Verification items for the finished model (mm, model axes). A direction names the side the tool comes from. Coordinates: 2 decimals unless noted, no trailing zeros. Loops run counter-clockwise (first coordinate to the right, second up) from the corner with the lowest first, then second, coordinate; pieces in that order, holes last.
Q1. Access from +Z, -Z, +X, -X, +Y, -Y to the whole of each face (thin tool, end or side, straight path). Record for faces 5 (the face through (-64.31, -64, 1.48)), 6 (the face through (-85.8, -89, 4)), 7 (the face through (-63, -78, 4)), 8 (the face through (-61.7, -66.3, 3)), 9 (the face through (-60, -79, 4)).
Q2. Go/stop test with flat-tipped pins: P1, Ø1.5, axis at x = -74, z = 6.5, coming from the +Y side; P2, Ø1.5, axis at x = -61.5, z = 6, coming from the +Y side; P3, Ø1.7, axis at y = -88.5, z = 4.5, coming from the -X side. Record where each tip stops, or that it passes through.
Q3. Sectioned sample at C-C (x = -69). Enter the section's corners in (y, z).
Q4. Mould release check, pull along Y, two halves, no side actions. Record for faces 1 (the face through (-62, -62, 1)), 2 (the face through (-66, -65, 1)), 3 (the face through (-75, -90, 4)), 4 (the face through (-87, -88.5, 2.4)): +Y half, -Y half, draft (parallel to the pull), parting line (faces both ways), or undercut.
Q5. Sectioned sample at B-B (z = 1.75). Enter the section's corners in (x, y).
Q6. Sectioned sample at A-A (y = -65). Enter the section's corners in (x, z), then the cut area to 3 significant figures.
Q7. Material ranges on probe 1 along X at (y, z) = (-65, 1.5); probe 2 along Y at (x, z) = (-64.5, 1.25); probe 3 along X at (y, z) = (-85.5, 3.25), recorded low to high.
Q8. Sectioned sample at D-D (y = -71). Enter the section's corners in (x, z), then the cut area to 3 significant figures.
Autodesk Inventor part; units mm, degrees
ref_plane "YZ Plane" through (0, 0, 0) normal (1, 0, 0) x (0, 1, 0)
ref_plane "XZ Plane" through (0, 0, 0) normal (0, 1, 0) x (-1, 0, 0)
ref_plane "XY Plane" through (0, 0, 0) normal (0, 0, 1) x (1, 0, 0)
sketch "Sketch1" plane through (0, 0, 0) normal (0, 0, 1) x (1, 0, 0)
  line L0 (-58, -60) -> (-60, -60)
  line L1 (-60, -60) -> (-60, -39.5)
  line L2 (-60, -39.5) -> (-58, -39.5)
  line L3 (-58, -39.5) -> (-58, -60)
  line L4 (49.6, 30) -> (51.6, 30)
  line L5 (51.6, 30) -> (51.6, 9.5)
  line L6 (51.6, 9.5) -> (49.6, 9.5)
  line L7 (49.6, 9.5) -> (49.6, 30)
  line L8 (-58, 39.5) -> (-60, 39.5)
  line L9 (-60, 39.5) -> (-60, 60)
  line L10 (-60, 60) -> (-58, 60)
  line L11 (-58, 60) -> (-58, 39.5)
  line L12 (-21.6, -39.5) -> (-19.6, -39.5)
  line L13 (-19.6, -39.5) -> (-19.6, -60)
  line L14 (-19.6, -60) -> (-21.6, -60)
  line L15 (-21.6, -60) -> (-21.6, -39.5)
  line L16 (51.6, -30) -> (49.6, -30)
  line L17 (49.6, -30) -> (49.6, -9.5)
  line L18 (49.6, -9.5) -> (51.6, -9.5)
  line L19 (51.6, -9.5) -> (51.6, -30)
  line L20 (-21.6, 60) -> (-19.6, 60)
  line L21 (-19.6, 60) -> (-19.6, 39.5)
  line L22 (-19.6, 39.5) -> (-21.6, 39.5)
  line L23 (-21.6, 39.5) -> (-21.6, 60)
  line L24 (90, -35) -> (90, 35)
  line L25 (90, 35) -> (49.6, 35)
  line L26 (49.6, 35) -> (49.6, 60)
  line L27 (49.6, 60) -> (90, 60)
  line L28 (90, 60) -> (90, 90)
  line L29 (90, 90) -> (-19.6, 90)
  line L30 (-19.6, 90) -> (-19.6, 65)
  line L31 (-19.6, 65) -> (-60, 65)
  line L32 (-60, 65) -> (-60, 90)
  line L33 (-60, 90) -> (-90, 90)
  line L34 (-90, 90) -> (-90, -90)
  line L35 (-90, -90) -> (-60, -90)
  line L36 (-60, -90) -> (-60, -65)
  line L37 (-60, -65) -> (-19.6, -65)
  line L38 (-19.6, -65) -> (-19.6, -90)
  line L39 (-19.6, -90) -> (90, -90)
  line L40 (90, -90) -> (90, -60)
  line L41 (90, -60) -> (49.6, -60)
  line L42 (49.6, -60) -> (49.6, -35)
  line L43 (49.6, -35) -> (90, -35)
  line L44 (86, -32) -> (73.8, -32)
  line L45 (73.8, -32) -> (73.8, -7.5)
  line L46 (73.8, -7.5) -> (86, -7.5)
  line L47 (86, -7.5) -> (86, -32)
  line L48 (65.8, -32) -> (53.6, -32)
  line L49 (53.6, -32) -> (53.6, -7.5)
  line L50 (53.6, -7.5) -> (65.8, -7.5)
  line L51 (65.8, -7.5) -> (65.8, -32)
  line L52 (86, -86) -> (70.6, -86)
  line L53 (70.6, -86) -> (70.6, -69.8)
  line L54 (70.6, -69.8) -> (86, -69.8)
  line L55 (86, -69.8) -> (86, -86)
  line L56 (86, 86) -> (86, 69.8)
  line L57 (86, 69.8) -> (70.6, 69.8)
  line L58 (70.6, 69.8) -> (70.6, 86)
  line L59 (70.6, 86) -> (86, 86)
  line L60 (73.8, 32) -> (86, 32)
  line L61 (86, 32) -> (86, 7.5)
  line L62 (86, 7.5) -> (73.8, 7.5)
  line L63 (73.8, 7.5) -> (73.8, 32)
  line L64 (65.8, 32) -> (65.8, 7.5)
  line L65 (65.8, 7.5) -> (53.6, 7.5)
  line L66 (53.6, 7.5) -> (53.6, 32)
  line L67 (53.6, 32) -> (65.8, 32)
  line L68 (-69.6, -87) -> (-85, -87)
  line L69 (-85, -87) -> (-85, -70.8)
  line L70 (-85, -70.8) -> (-69.6, -70.8)
  line L71 (-69.6, -70.8) -> (-69.6, -87)
  line L72 (-56, -62) -> (-56, -37.5)
  line L73 (-56, -37.5) -> (-43.8, -37.5)
  line L74 (-43.8, -37.5) -> (-43.8, -62)
  line L75 (-43.8, -62) -> (-56, -62)
  line L76 (-56, 62) -> (-43.8, 62)
  line L77 (-43.8, 62) -> (-43.8, 37.5)
  line L78 (-43.8, 37.5) -> (-56, 37.5)
  line L79 (-56, 37.5) -> (-56, 62)
  line L80 (-23.6, 62) -> (-23.6, 37.5)
  line L81 (-23.6, 37.5) -> (-35.8, 37.5)
  line L82 (-35.8, 37.5) -> (-35.8, 62)
  line L83 (-35.8, 62) -> (-23.6, 62)
  line L84 (-23.6, -62) -> (-35.8, -62)
  line L85 (-35.8, -62) -> (-35.8, -37.5)
  line L86 (-35.8, -37.5) -> (-23.6, -37.5)
  line L87 (-23.6, -37.5) -> (-23.6, -62)
  line L88 (-85, 87) -> (-69.6, 87)
  line L89 (-69.6, 87) -> (-69.6, 70.8)
  line L90 (-69.6, 70.8) -> (-85, 70.8)
  line L91 (-85, 70.8) -> (-85, 87)
  line L92 (-63, -68) -> (-60, -68)
  line L93 (-60, -68) -> (-60, -65)
  line L94 (-60, -65) -> (-19.6, -65)
  line L95 (-90, -90) -> (-60, -90)
  line L96 (-60, -90) -> (-60, -87)
  line L97 (-60, -87) -> (-90, -87)
  line L98 (-90, -87) -> (-90, -90)
  line L99 (-60, -87) -> (-63, -87)
  line L100 (-63, -87) -> (-63, -68)
  line L101 (-63, -68) -> (-60, -68)
  line L102 (-60, -68) -> (-60, -87)
  line L103 (-60, -68) -> (-66, -68)
  line L104 (-66, -68) -> (-66, -62)
  line L105 (-66, -62) -> (-60, -62)
  line L106 (-60, -62) -> (-60, -68)
  circle A0 centre (-63, -65) radius 1.5
  circle A1 centre (-16.6, -87) radius 1.5
  circle A2 centre (49.6, -87) radius 1.5
  circle A3 centre (46.6, -60) radius 1.5
  circle A4 centre (87, -63) radius 1.5
  circle A5 centre (46.6, -32) radius 1.5
  circle A6 centre (46.6, 32) radius 1.5
  circle A7 centre (87, 63) radius 1.5
  circle A8 centre (46.6, 60) radius 1.5
  circle A9 centre (49.6, 87) radius 1.5
  circle A10 centre (-16.6, 87) radius 1.5
  circle A11 centre (-16.6, 65) radius 1.5
  circle A12 centre (-63, 65) radius 1.5
  arc A13 (-63, -62) -> (-63, -68) centre (-63, -65) ccw
  arc A14 (-16.6, -68) -> (-16.6, -62) centre (-16.6, -65) ccw
  line L107 (-16.6, -62) -> (-63, -62)
  line L108 (-76, -39.25) -> (-82, -39.25)
  line L109 (-82, -39.25) -> (-82, -20.75)
  line L110 (-82, -20.75) -> (-76, -20.75)
  line L111 (-76, -20.75) -> (-76, -39.25)
  line L112 (-76, 20.75) -> (-82, 20.75)
  line L113 (-82, 20.75) -> (-82, 39.25)
  line L114 (-82, 39.25) -> (-76, 39.25)
  line L115 (-76, 39.25) -> (-76, 20.75)
  line L116 (-19.6, -68) -> (-16.6, -68)
  circle A15 centre (-86.5, -55.7158) radius 1.25
  circle A16 centre (-86.5, 55.8) radius 1.25
  circle A17 centre (-79.5, -5.4579) radius 1.25
  circle A18 centre (-79.5, 5.5421) radius 1.25
  line L117 (-19.6, -65) -> (-19.6, -68)
  point P0 (0, 0)
  dimension "d0" = 3
extrude "Extrusion1" add sketch "Sketch1" along normal blind 8 contours L36 L97 L100 L92 | L36 L35 L34 L97 L68
ref_plane "Work Plane1" through (0, 0, 0) normal (0, 0, 1) x (1, 0, 0)
sketch "Sketch2" plane through (0, 0, 0) normal (0, 0, 1) x (1, 0, 0)
  line L0 (-63, -68) -> (-60, -68)
  line L1 (-60, -68) -> (-60, -65)
  line L2 (-60, -65) -> (-19.6, -65)
  circle A0 centre (-63, -65) radius 2
  line L3 (-60, -90) -> (-60, -68)
  line L4 (-60, -68) -> (-66, -68)
  line L5 (-66, -68) -> (-66, -62)
  line L6 (-66, -62) -> (-60, -62)
  line L7 (-60, -62) -> (-60, -68)
  circle A1 centre (-63, -65) radius 1.65
  arc A2 (-63, -62) -> (-63, -68) centre (-63, -65) ccw
  arc A3 (-16.6, -68) -> (-16.6, -62) centre (-16.6, -65) ccw
  line L8 (-16.6, -62) -> (-63, -62)
  line L9 (-19.6, -68) -> (-16.6, -68)
  line L10 (-19.6, -65) -> (-19.6, -68)
  point P0 (0, 0)
  dimension "d3" = 3.3
extrude "Extrusion2" add sketch "Sketch2" along normal blind 3 contours A2 L6 L7 L1 L0 | A0
sketch "Sketch3" plane through (-90, -90, 0) normal (0, -1, 0) x (1, 0, 0)
  line L0 (0, 0) -> (0, 8)
  line L1 (0, 3.137) -> (9.9706, 8)
  line L2 (0, 3.137) -> (11.0933, 3.137) construction
  line L3 (0, 8) -> (30, 8)
  point P0 (90, 0)
  dimension "d7" = 26
  dimension "d8" = 3.137
extrude "Extrusion3" cut sketch "Sketch3" against normal blind 3
sketch "Sketch4" plane through (-90, -90, 0) normal (0, -1, 0) x (1, 0, 0)
  circle A0 centre (3, 3.6) radius 1.2
  line L0 (1.8, 2.4) -> (4.2, 2.4)
  line L1 (4.2, 2.4) -> (4.2, 4.8)
  line L2 (4.2, 4.8) -> (1.8, 4.8)
  line L3 (1.8, 4.8) -> (1.8, 2.4)
  line L4 (1.8, 2.4) -> (4.2, 4.8) construction
  line L5 (4.2, 2.4) -> (1.8, 4.8) construction
  line L6 (4.2, 4.8) -> (4.2, 5.1855)
  line L7 (0, 3.137) -> (9.9706, 8)
  line L8 (4.2, 5.1855) -> (3, 4.6002)
  point P0 (90, 0)
  point P1 (1.8, 4.0149)
  point P2 (1.8, 3.6)
  point P3 (4.2, 3.6)
extrude "Extrusion4" cut sketch "Sketch4" against normal blind 3 contours A0 L7 | A0 L7 L2 L1 | L2 L7 L6 | L3 L7 A0 picked at (3.089, 3.1434)
properties part number "rightfrontwall"
Geometry check:
1. face 5: +Z, -Z
1. face 6: +Z, +Y, -Y
1. face 7: +Z, -Z, -X
1. face 8: +Z, +X, -X, +Y
1. face 9: +Z, -Z, +X, +Y, -Y
2. P1: stops at y = -87
2. P2: stops at y = -68
2. P3: stops at x = -88.95
3. outline: (-90, 0) - (-87, 0) - (-87, 8) - (-90, 8) - close
4. face 1: +Y half
4. face 2: undercut
4. face 3: -Y half
4. face 4: draft
5. outline: (-90, -90) - (-60, -90) - (-60, -62) - (-63, -62) arc R3 ccw to (-63, -68) - (-63, -87) - (-90, -87) - close; hole circle Ø3.3 at (-63, -65)
6. outline: (-66, 0) - (-64.65, 0) - (-64.65, 3) - (-66, 3) - close; (-61.35, 0) - (-60, 0) - (-60, 3) - (-61.35, 3) - close
6. area: 8.10 mm2
7. probe 1: x = -66 to -64.65, -61.35 to -60
7. probe 2: y = -90 to -87, -67.6 to -65.69, -64.31 to -62.4
7. probe 3: x = -63 to -60
8. outline: (-63, 0) - (-60, 0) - (-60, 8) - (-63, 8) - close
8. area: 24.0 mm2
